The listing builds one solid part. Answer for the finished solid, in the listing's coordinates (mm). Give positions to 0.01 mm unless a question says otherwise; leave off trailing zeros. Loops run counter-clockwise (first coordinate to the right, second up) from the corner with the lowest first, then second, coordinate; pieces in that order, holes last. Notation, with made-up numbers: (22, -19) - (76, -19) arc R29 cw to (76, 9) - close; hole circle Ø5 at (86.25, 26). An arc over 180 degrees is marked (long way). Write item = value, one per line. Start each with the question number.
1) A flat-ended cylindrical pin translates along its axis: P1, Ø8, axis at x = 50, z = -50, coming from the +Y side. Find the tip coordinate at first contact, or state that the pin passes through.
2) The part is cut by section B-B on z = 50. Write down the section's boundary in (x, y), plus the area to 3 significant figures.
3) The mould has two halves that part along X. Classify faces 1 (the cylindrical face through (54.957, 6.084, 49.349)), 2 (the flat face through (-97, 6, -98)), 3 (the flat face through (-1, 0, -1)): +X half, -X half, draft (parallel to the pull), parting line (faces both ways), or undercut.
4) Consider probe 1 along X at (y, z) = (3.25, 50). Determine where the line is inside the solid, lowest interval first.
5) The part is cut by section A-A on x = -50. Write down the section's boundary in (y, z).
from build123d import *

# Parameters (mm, degrees)
SKETCH1_W           = 200
SKETCH1_H           = 200
BOSS_EXTRUDE1_DEPTH = 12
CUT_EXTRUDE2_REACH  = 143.93
SKETCH3_R           = 5
CHAMFER1_SIZE       = 5


with BuildPart() as part:
    # Sketch1 → Boss-Extrude1 (new body)
    with BuildSketch(Plane(origin=(0, 0, 0), x_dir=(1, 0, 0), z_dir=(0, 1, 0))):
        Rectangle(SKETCH1_W, SKETCH1_H)
    extrude(amount=BOSS_EXTRUDE1_DEPTH)

    # Sketch3 → Cut-Extrude2 (cut, up to next)
    with BuildSketch(Plane(origin=(0, 12, 0), x_dir=(1, 0, 0), z_dir=(0, 1, 0)), mode=Mode.PRIVATE) as cut_extrude2_sk1:
        with Locations(Location((-50, 50, 0), (0, 0, 270))):
            Circle(SKETCH3_R)
    cut_extrude2_tool1 = extrude(cut_extrude2_sk1.sketch, amount=-CUT_EXTRUDE2_REACH, mode=Mode.PRIVATE) & part.part
    # Sketch3 → Cut-Extrude2 (cut, up to next)
    with BuildSketch(Plane(origin=(0, 12, 0), x_dir=(1, 0, 0), z_dir=(0, 1, 0)), mode=Mode.PRIVATE) as cut_extrude2_sk2:
        with Locations(Location((50, 50, 0), (0, 0, 270))):
            Circle(SKETCH3_R)
    cut_extrude2_tool2 = extrude(cut_extrude2_sk2.sketch, amount=-CUT_EXTRUDE2_REACH, mode=Mode.PRIVATE) & part.part
    # Sketch3 → Cut-Extrude2 (cut, up to next)
    with BuildSketch(Plane(origin=(0, 12, 0), x_dir=(1, 0, 0), z_dir=(0, 1, 0)), mode=Mode.PRIVATE) as cut_extrude2_sk3:
        with Locations(Location((-50, -50, 0), (0, 0, 270))):
            Circle(SKETCH3_R)
    cut_extrude2_tool3 = extrude(cut_extrude2_sk3.sketch, amount=-CUT_EXTRUDE2_REACH, mode=Mode.PRIVATE) & part.part
    # Sketch3 → Cut-Extrude2 (cut, up to next)
    with BuildSketch(Plane(origin=(0, 12, 0), x_dir=(1, 0, 0), z_dir=(0, 1, 0)), mode=Mode.PRIVATE) as cut_extrude2_sk4:
        with Locations(Location((50, -50, 0), (0, 0, 270))):
            Circle(SKETCH3_R)
    cut_extrude2_tool4 = extrude(cut_extrude2_sk4.sketch, amount=-CUT_EXTRUDE2_REACH, mode=Mode.PRIVATE) & part.part
    add(cut_extrude2_tool1.solids().sort_by_distance((-50, 12, -50))[0], mode=Mode.SUBTRACT)
    add(cut_extrude2_tool2.solids().sort_by_distance((50, 12, -50))[0], mode=Mode.SUBTRACT)
    add(cut_extrude2_tool3.solids().sort_by_distance((-50, 12, 50))[0], mode=Mode.SUBTRACT)
    add(cut_extrude2_tool4.solids().sort_by_distance((50, 12, 50))[0], mode=Mode.SUBTRACT)

    # Chamfer1
    chamfer1_edges = [part.edges().sort_by_distance(p)[0] for p in [
        (-100, 6, -100),
        (100, 6, -100),
        (100, 6, 100),
        (-100, 6, 100),
    ]]
    chamfer(chamfer1_edges, length=CHAMFER1_SIZE)


solid = part.part
Answer below:
q1.P1 = through
q2.outline = (-100, 0) - (-55, 0) - (-55, 12) - (-100, 12) - close; (-45, 0) - (45, 0) - (45, 12) - (-45, 12) - close; (55, 0) - (100, 0) - (100, 12) - (55, 12) - close
q2.area = 2,160 mm2
q3.face_1 = undercut
q3.face_2 = -X half
q3.face_3 = draft
q4.probe_1 = -100 to -55, -45 to 45, 55 to 100
q5.outline = (0, -100) - (12, -100) - (12, -55) - (0, -55) - close; (0, -45) - (12, -45) - (12, 45) - (0, 45) - close; (0, 55) - (12, 55) - (12, 100) - (0, 100) - close
